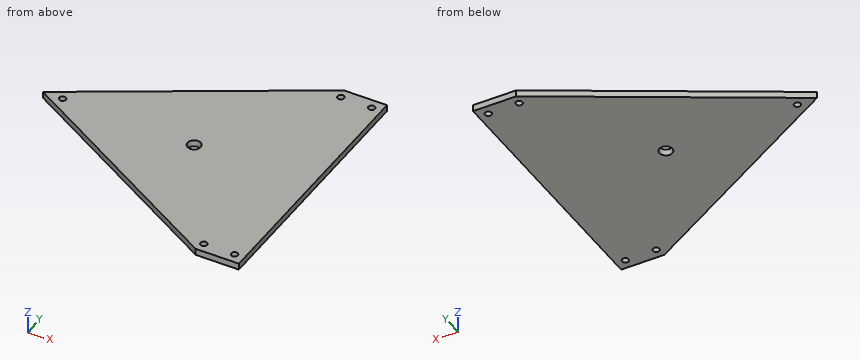
from build123d import *

# Parameters (mm, degrees)
SKETCH1_R           = 2.5
SKETCH1_R_2         = 5
BOSS_EXTRUDE1_DEPTH = 5


with BuildPart() as part:
    # Sketch1 → Boss-Extrude1 (new body)
    with BuildSketch(Plane.XY):
        Polygon((-30.5, 0), (-203.705080757, -100), (-30.5, -200), (2.5, -200), (2.5, 0), align=None)
        with Locations((-188.705080757, -100)):
            Circle(SKETCH1_R, mode=Mode.SUBTRACT)
        with Locations((-28.490381057, -7.5)):
            Circle(SKETCH1_R, mode=Mode.SUBTRACT)
        with Locations((-5, -7.5)):
            Circle(SKETCH1_R, mode=Mode.SUBTRACT)
        with Locations((-5, -192.5)):
            Circle(SKETCH1_R, mode=Mode.SUBTRACT)
        with Locations((-28.490381057, -192.5)):
            Circle(SKETCH1_R, mode=Mode.SUBTRACT)
        with Locations((-87.586729605, -101.122883886)):
            Circle(SKETCH1_R_2, mode=Mode.SUBTRACT)
    extrude(amount=BOSS_EXTRUDE1_DEPTH)


solid = part.part
Geometry check sheet. Reference: the model listing, model coordinates, mm. Give positions to 0.01 mm unless a question says otherwise; leave off trailing zeros. Write each loop counter-clockwise with the first axis right and the second up, starting at its lowest first coordinate (ties: lowest second). Pieces come first, ordered by that corner, then holes.
1) Cross-section at D-D (y = -161). Record the boundary of the cut face in (x, z).
Values follow:
outline: (-98.05, 0) - (2.5, 0) - (2.5, 5) - (-98.05, 5) - close
2) Cross-section at C-C (z = 4). Record the boundary of the cut face in (x, y), plus the area to 3 significant figures.
Values follow:
outline: (-203.71, -100) - (-30.5, -200) - (2.5, -200) - (2.5, 0) - (-30.5, 0) - close; hole circle Ø5 at (-188.71, -100); hole circle Ø10 at (-87.59, -101.12); hole circle Ø5 at (-28.49, -192.5); hole circle Ø5 at (-28.49, -7.5); hole circle Ø5 at (-5, -192.5); hole circle Ø5 at (-5, -7.5)
area: 23,700 mm2
3) Go/stop test with flat-tipped pins: pin 1 Ø8 at (x, y) = (-87.59, -101.12) entering from -Z; pin 2 Ø4 at (x, y) = (-178, -103) entering from -Z; pin 3 Ø2 at (y, z) = (-173.5, 2) entering from -X; pin 4 Ø1 at (x, z) = (-88.5, 3) entering from -Y. Record where each tip stops, or that it passes through.
Values follow:
pin 1: passes through
pin 2: stops at z = 0
pin 3: stops at x = -78.13
pin 4: stops at y = -166.8
4) Cross-section at A-A (x = -5). Record the boundary of the cut face in (y, z).
Values follow:
outline: (-200, 0) - (-195, 0) - (-195, 5) - (-200, 5) - close; (-190, 0) - (-10, 0) - (-10, 5) - (-190, 5) - close; (-5, 0) - (0, 0) - (0, 5) - (-5, 5) - close
5) Thickness scan on line 1 (Y direction, x = -5, z = 3.2); line 2 (Y direction, x = -85.5, z = 3.5); line 3 (X direction, y = -59.5, z = 1.85). Record the ranges inside material, lowest first.
Values follow:
line 1: y = -200 to -195, -190 to -10, -5 to 0
line 2: y = -168.25 to -105.67, -96.58 to -31.75
line 3: x = -133.56 to 2.5
6) Cross-section at B-B (y = -7.5). Record the boundary of the cut face in (x, z).
Values follow:
outline: (-43.49, 0) - (-30.99, 0) - (-30.99, 5) - (-43.49, 5) - close; (-25.99, 0) - (-7.5, 0) - (-7.5, 5) - (-25.99, 5) - close; (-2.5, 0) - (2.5, 0) - (2.5, 5) - (-2.5, 5) - close
